Read the model definition and answer for the solid it produces. Units are mm, in the model's axes. A direction names the side the tool comes from. Round coordinates to 2 decimals unless told otherwise and drop trailing zeros. Write each loop counter-clockwise with the first axis right and the second up, starting at its lowest first coordinate (ties: lowest second). Pieces come first, ordered by that corner, then holes. Notation, with made-up numbers: (33, 34.25) -> (89, 34.25) arc R24 cw to (89, 70.25) -> close; hole circle Ø1 at (-32, -39). An arc over 180 degrees is marked (long way). Return JSON: item names as keys, results as strings.
from build123d import *

# Parameters (mm, degrees)
BOSS_EXTRUDE1_DEPTH = 8
SKETCH7_W           = 30
SKETCH7_H           = 15.4
BOSS_EXTRUDE2_DEPTH = 40
SKETCH8_W           = 30
SKETCH8_H           = 10
BOSS_EXTRUDE3_DEPTH = 19.1
SKETCH9_R           = 8
CUT_EXTRUDE1_DEPTH  = 10
FILLET2_R           = 15
FILLET3_R           = 5
SKETCH11_R          = 7.5
CUT_EXTRUDE2_DEPTH  = 38
SKETCH14_W          = 8
SKETCH14_H          = 5
BOSS_EXTRUDE5_DEPTH = 8
SKETCH15_W          = 48
SKETCH15_H          = 5
BOSS_EXTRUDE6_DEPTH = 8
SKETCH16_R          = 2.15
CUT_EXTRUDE4_DEPTH  = 5


with BuildPart() as part:
    # Sketch6 → Boss-Extrude1 (new body)
    with BuildSketch(Plane.XY):
        Polygon((-16.08404704, 11.385723939), (-16.08404704, -7.714276061), (24.31595296, -7.714276061), (24.31595296, 11.385723939), (34.31595296, 11.385723939), (34.31595296, -23.114276061), (-26.08404704, -23.114276061), (-26.08404704, 11.385723939), align=None)
        with BuildLine():
            Line((-19.83404704, 4.635723939), (-21.33404704, 4.635723939))
            ThreePointArc((-21.33404704, 4.635723939), (-23.58404704, 6.885723939), (-21.33404704, 9.135723939))
            Line((-21.33404704, 9.135723939), (-19.83404704, 9.135723939))
            ThreePointArc((-19.83404704, 9.135723939), (-17.58404704, 6.885723939), (-19.83404704, 4.635723939))
        make_face(mode=Mode.SUBTRACT)
        with BuildLine():
            Line((-19.83404704, -5.364276061), (-21.33404704, -5.364276061))
            ThreePointArc((-21.33404704, -5.364276061), (-23.58404704, -3.114276061), (-21.33404704, -0.864276061))
            Line((-21.33404704, -0.864276061), (-19.83404704, -0.864276061))
            ThreePointArc((-19.83404704, -0.864276061), (-17.58404704, -3.114276061), (-19.83404704, -5.364276061))
        make_face(mode=Mode.SUBTRACT)
        with BuildLine():
            Line((28.06595296, -5.364276061), (29.56595296, -5.364276061))
            ThreePointArc((29.56595296, -5.364276061), (31.81595296, -3.114276061), (29.56595296, -0.864276061))
            Line((29.56595296, -0.864276061), (28.06595296, -0.864276061))
            ThreePointArc((28.06595296, -0.864276061), (25.81595296, -3.114276061), (28.06595296, -5.364276061))
        make_face(mode=Mode.SUBTRACT)
        with BuildLine():
            Line((28.06595296, 4.635723939), (29.56595296, 4.635723939))
            ThreePointArc((29.56595296, 4.635723939), (31.81595296, 6.885723939), (29.56595296, 9.135723939))
            Line((29.56595296, 9.135723939), (28.06595296, 9.135723939))
            ThreePointArc((28.06595296, 9.135723939), (25.81595296, 6.885723939), (28.06595296, 4.635723939))
        make_face(mode=Mode.SUBTRACT)
    extrude(amount=BOSS_EXTRUDE1_DEPTH)

    # Sketch7 → Boss-Extrude2 (add)
    with BuildSketch(Plane.XY.offset(8)):
        with Locations((-11.08404704, -15.414276061)):
            Rectangle(SKETCH7_W, SKETCH7_H)
    extrude(amount=BOSS_EXTRUDE2_DEPTH)

    # Sketch8 → Boss-Extrude3 (add)
    with BuildSketch(Plane(origin=(0, -7.714276061, 0), x_dir=(1, 0, 0), z_dir=(0, 1, 0))):
        with Locations((-11.08404704, -43)):
            Rectangle(SKETCH8_W, SKETCH8_H)
    extrude(amount=BOSS_EXTRUDE3_DEPTH)

    # Sketch9 → Cut-Extrude1 (cut)
    with BuildSketch(Plane.XY.offset(48)):
        with Locations((-6.88404704, 1.885723939)):
            Circle(SKETCH9_R)
    extrude(amount=-CUT_EXTRUDE1_DEPTH, mode=Mode.SUBTRACT)

    # Fillet2
    fillet2_edges = [part.edges().sort_by_distance(p)[0] for p in [
        (-26.08404704, 11.385723939, 43),
    ]]
    fillet(fillet2_edges, radius=FILLET2_R)

    # Fillet3
    fillet3_edges = [part.edges().sort_by_distance(p)[0] for p in [
        (3.91595296, 11.385723939, 43),
    ]]
    fillet(fillet3_edges, radius=FILLET3_R)

    # Sketch11 → Cut-Extrude2 (cut)
    with BuildSketch(Plane(origin=(0, 0, 0), x_dir=(-1, 0, 0), z_dir=(0, 0, -1))):
        with Locations((6.88404704, -2.044839291)):
            Circle(SKETCH11_R)
    extrude(amount=-CUT_EXTRUDE2_DEPTH, mode=Mode.SUBTRACT)

    # Sketch14 → Boss-Extrude5 (add)
    with BuildSketch(Plane(origin=(34.31595296, 0, 0), x_dir=(0, 0, -1), z_dir=(1, 0, 0))):
        with Locations((-4, -20.614276061)):
            Rectangle(SKETCH14_W, SKETCH14_H)
    extrude(amount=BOSS_EXTRUDE5_DEPTH)

    # Sketch15 → Boss-Extrude6 (add)
    with BuildSketch(Plane.ZY.offset(26.08404704)):
        with Locations((24, -20.614276061)):
            Rectangle(SKETCH15_W, SKETCH15_H)
    extrude(amount=BOSS_EXTRUDE6_DEPTH)

    # Sketch16 → Cut-Extrude4 (cut)
    with BuildSketch(Plane(origin=(0, -18.114276061, 0), x_dir=(1, 0, 0), z_dir=(0, 1, 0))):
        with Locations((-30.08404704, -11)):
            Circle(SKETCH16_R)
        with Locations((-30.08404704, -36)):
            Circle(SKETCH16_R)
        with Locations((38.31595296, -4)):
            Circle(SKETCH16_R)
    extrude(amount=-CUT_EXTRUDE4_DEPTH, mode=Mode.SUBTRACT)


solid = part.part
Item 1: Straight lines are drawn through the part: L1, parallel to Z at x = -17, y = -3.5; L2, parallel to X at y = -19.4, z = 36; L3, parallel to X at y = -21.2, z = 4. For each, find the intervals that lie inside material, in ascending order. Write a range as [from, to].
Worked answers:
{"L1": "z = [0, 8], [38, 48]", "L2": "x = [-34.08, -32.23], [-27.93, 3.92]", "L3": "x = [-34.08, 36.17], [40.47, 42.32]"}
Item 2: Section B-B (y = -20) is taken. Give the vertices of the cut face in (x, z).
Worked answers:
{"outline": "(-34.08, 0) -> (42.32, 0) -> (42.32, 8) -> (3.92, 8) -> (3.92, 48) -> (-34.08, 48) -> close; hole circle Ø4.3 at (-30.08, 11); hole circle Ø4.3 at (-30.08, 36); hole circle Ø4.3 at (38.32, 4)"}
Item 3: For a pull along Y with two mould halves and no side action, classify faces 1 (the flat face through (29, -0.864, 4)), 2 (the flat face through (-11, -10, 48)), 3 (the cylindrical face through (-23.584, 6.836, 3.944)), 4 (the cylindrical face through (2.41, 9.96, 42.93)) as released by +Y, released by -Y, zero draft, split by the parting line, or undercut.
Worked answers:
{"face 1": "undercut", "face 2": "zero draft", "face 3": "undercut", "face 4": "released by +Y"}
Item 4: Section D-D (y = -2) is taken. Give the vertices of the cut face in (x, z), then the cut area to 3 significant figures.
Worked answers:
{"outline": "(-26.08, 0) -> (-23.29, 0) -> (-23.29, 8) -> (-26.08, 8) -> close; (-26, 38) -> (-13.88, 38) -> (-13.88, 48) -> (-26, 48) -> close; (-17.88, 0) -> (-16.08, 0) -> (-16.08, 8) -> (-17.88, 8) -> close; (0.11, 38) -> (3.92, 38) -> (3.92, 48) -> (0.11, 48) -> close; (24.32, 0) -> (26.11, 0) -> (26.11, 8) -> (24.32, 8) -> close; (31.52, 0) -> (34.32, 0) -> (34.32, 8) -> (31.52, 8) -> close", "area": "233 mm2"}
Item 5: Section C-C (z = 4) is taken. State how many separate pieces and enclosed holes the cut face has, then the cut area to 3 significant figures.
Worked answers:
{"separate pieces": "2", "enclosed holes": "4", "area": "1,270 mm2"}
Item 6: Section A-A (z = 11) is taken. Give the vertices of the cut face in (x, y).
Worked answers:
{"outline": "(-34.08, -23.11) -> (-32.23, -23.11) -> (-32.23, -18.11) -> (-34.08, -18.11) -> close; (-27.93, -23.11) -> (3.92, -23.11) -> (3.92, -7.71) -> (-1.97, -7.71) arc R7.5 cw to (-11.79, -7.71) -> (-26.08, -7.71) -> (-26.08, -18.11) -> (-27.93, -18.11) -> close"}
Item 7: A tool of negligible diameter and unlimited length cuts with its end or side. For faces 5 (the flat face through (-21, -5.364, 4)), 6 (the cylindrical face through (-21.807, 6.875, 42.93)), 7 (the flat face through (-21, 9.136, 4)), 8 (the flat face through (24.316, 2, 4)), from which of +Z, -Z, +X, -X, +Y, -Y can it reach the whole face along a straight path? Write none if from no direction.
Worked answers:
{"face 5": "-Z", "face 6": "+Z, -X, +Y", "face 7": "+Z, -Z", "face 8": "+Z, -Z, +Y"}
Item 8: Flat-ended cylindrical pins translate along their axes: pin 1 (2.5 mm diameter, centred on y = 1.5, z = 5, fed in from +X); pin 2 (4 mm diameter, centred on x = -28.5, z = 31, fed in from +Y); pin 3 (7 mm diameter, centred on x = -20.5, z = 26, fed in from +Y). Find the tip coordinate at first contact, or state that the pin passes through.
Worked answers:
{"pin 1": "stops at x = 34.32", "pin 2": "stops at y = -18.11", "pin 3": "stops at y = -7.71"}
